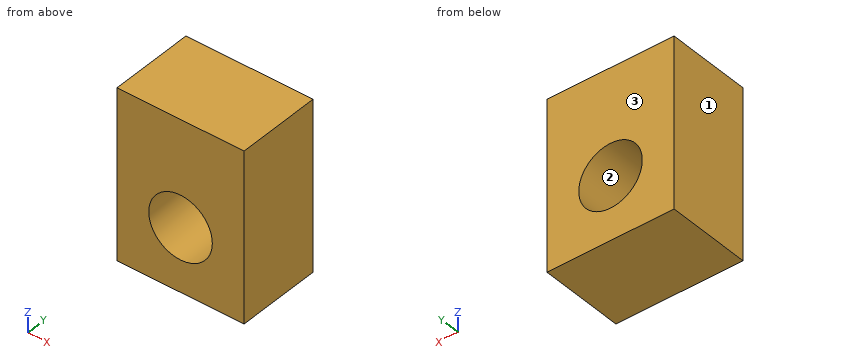
Autodesk Inventor part; units mm, degrees
ref_plane "YZ Plane" through (0, 0, 0) normal (1, 0, 0) x (0, 1, 0)
ref_plane "XZ Plane" through (0, 0, 0) normal (0, 1, 0) x (-1, 0, 0)
ref_plane "XY Plane" through (0, 0, 0) normal (0, 0, 1) x (1, 0, 0)
sketch "Sketch1" plane through (0, 0, 0) normal (0, 1, 0) x (-1, 0, 0)
  line L0 (15, 20) -> (-15, 20)
  line L1 (-15, 20) -> (-15, -20)
  line L2 (-15, -20) -> (15, -20)
  line L3 (15, -20) -> (15, 20)
  point P0 (0, 0)
  point P1 (15, 0)
  point P2 (0, -20)
  dimension "d0" = 40
  dimension "d1" = 30
extrude "Extrusion1" add sketch "Sketch1" along normal blind 20
sketch "Sketch2" plane through (0, 20, 0) normal (0, 1, 0) x (1, 0, 0)
  circle A0 centre (0, 5) radius 7.5
  line L0 (15, 20) -> (-15, 20)
  point P0 (0, 0)
  point P1 (0, 20)
  dimension "d7" = 15
  dimension "d10" = 15
extrude "Extrusion2" cut sketch "Sketch2" against normal blind 20
properties part number "Slider"
The listing builds one solid part. Answer for the finished solid, in the listing's coordinates (mm). Face numbers are marked on the shaded views. Give positions to 0.01 mm unless a question says otherwise; leave off trailing zeros. Loops run counter-clockwise (first coordinate to the right, second up) from the corner with the lowest first, then second, coordinate; pieces in that order, holes last. Notation, with made-up numbers: M 2.5,-6.5 L 56.5,-6.5 A9 ccw 56.5,8.5 Z; hole C 52,63 d6. An arc over 180 degrees is marked long. One line per item, written item: value.
Q1. Determine the mould class of the marked faces 1, 2 and 3 for opening direction X: +X half, -X half, draft (parallel to the pull), parting line (faces both ways), or undercut.
Working result:
face 1: -X half
face 2: undercut
face 3: draft
Q2. A cutting plane is placed at C-C on y = 2.5. Determine the outline of the cut face in (x, z), then the cut area to 3 significant figures.
Working result:
outline: M -15,-20 L 15,-20 L 15,20 L -15,20 Z; hole C 0,-5 d15
area: 1,020 mm^2
Q3. A cutting plane is placed at B-B on x = 0. Determine the outline of the cut face in (y, z).
Working result:
outline: M 0,-20 L 20,-20 L 20,-12.5 L 0,-12.5 Z; M 0,2.5 L 20,2.5 L 20,20 L 0,20 Z
Q4. A cutting plane is placed at A-A on z = -5. Determine the outline of the cut face in (x, y), then the cut area to 3 significant figures.
Working result:
outline: M -15,0 L -7.5,0 L -7.5,20 L -15,20 Z; M 7.5,0 L 15,0 L 15,20 L 7.5,20 Z
area: 300 mm^2
Q5. Find the intervals of material crossed by line 1 (X direction, y = 4, z = -5); line 2 (Z direction, x = 0, y = 6); line 3 (Z direction, x = -1.5, y = 13), in increasing order. Write a range as from..to.
Working result:
line 1: x = -15..-7.5, 7.5..15
line 2: z = -20..-12.5, 2.5..20
line 3: z = -20..-12.35, 2.35..20
Q6. A flat-ended cylindrical pin translates along its axis: P1, Ø4, axis at x = -2, z = -10.5, coming from the -Y side. Find the tip coordinate at first contact, or state that the pin passes through.
Working result:
P1: stops at y = 0
